```python
from build123d import *

# Parameters (mm, degrees)
BOSS_EXTRU_1_DEPTH        = 13
COQUE1_T                  = -5
COQUE1_THICKNESS_2_FACE_W = 65
COQUE1_THICKNESS_2_FACE_H = 65
COQUE1_THICKNESS_2_DEPTH  = 2
ENL_V_MAT_EXTRU_1_REACH   = 88.587
ESQUISSE2_R               = 2.5
ENL_V_MAT_EXTRU_2_REACH   = 95.396
ESQUISSE3_R               = 2.5
BOSS_EXTRU_2_DEPTH        = 10


with BuildPart() as part:
    # Esquisse1 → Boss.-Extru.1 (new body)
    with BuildSketch(Plane.XY):
        Polygon((44.118436308, 33.728448276), (54.118436308, 33.728448276), (54.118436308, 23.728448276), (54.118436308, -41.271551724), (-20.881563692, -41.271551724), (-20.881563692, 33.728448276), align=None)
    extrude(amount=BOSS_EXTRU_1_DEPTH)

    # Coque1
    coque1_openings = [part.faces().sort_by_distance(p)[0] for p in [
        (16.618436308, -3.771551724, 13),
    ]]
    offset(amount=COQUE1_T, openings=coque1_openings, kind=Kind.INTERSECTION)

    # Coque1 thickness 2 face (on inner face of the shell) → Coque1 thickness 2 (cut)
    with BuildSketch(Plane(origin=(16.618436308, -3.771551724, 5), x_dir=(-1, 0, 0), z_dir=(0, 0, -1))):
        Rectangle(COQUE1_THICKNESS_2_FACE_W, COQUE1_THICKNESS_2_FACE_H)
    extrude(amount=COQUE1_THICKNESS_2_DEPTH, mode=Mode.SUBTRACT)

    # Enlèv. mat.-Extru.1: up to this face of the body (flat: up to its plane)
    enl_v_mat_extru_1_end = Plane(part.part.faces().sort_by_distance((54.118436308, -3.771551724, 6.5))[0])
    # Esquisse2 → Enlèv. mat.-Extru.1 (cut, up to the picked face)
    with BuildSketch(Plane.ZY.offset(20.881563692), mode=Mode.PRIVATE) as enl_v_mat_extru_1_sk1:
        with Locations(Location((8, -16.271551724, 0), (0, 0, 270))):
            Circle(ESQUISSE2_R)
    enl_v_mat_extru_1_tool1 = split(extrude(enl_v_mat_extru_1_sk1.sketch, amount=-ENL_V_MAT_EXTRU_1_REACH, mode=Mode.PRIVATE), bisect_by=enl_v_mat_extru_1_end, keep=Keep.BOTH, mode=Mode.PRIVATE)
    # Esquisse2 → Enlèv. mat.-Extru.1 (cut, up to the picked face)
    with BuildSketch(Plane.ZY.offset(20.881563692), mode=Mode.PRIVATE) as enl_v_mat_extru_1_sk2:
        with Locations(Location((8, 8.728448276, 0), (0, 0, 270))):
            Circle(ESQUISSE2_R)
    enl_v_mat_extru_1_tool2 = split(extrude(enl_v_mat_extru_1_sk2.sketch, amount=-ENL_V_MAT_EXTRU_1_REACH, mode=Mode.PRIVATE), bisect_by=enl_v_mat_extru_1_end, keep=Keep.BOTH, mode=Mode.PRIVATE)
    add(enl_v_mat_extru_1_tool1.solids().sort_by(Axis((-20.881564, -16.271552, 8), (1, 0, 0)))[0], mode=Mode.SUBTRACT)
    add(enl_v_mat_extru_1_tool2.solids().sort_by(Axis((-20.881564, 8.728448, 8), (1, 0, 0)))[0], mode=Mode.SUBTRACT)

    # Enlèv. mat.-Extru.2: up to this face of the body (flat: up to its plane)
    enl_v_mat_extru_2_end = Plane(part.part.faces().sort_by_distance((16.618436308, 33.728448276, 6.5))[0])
    # Esquisse3 → Enlèv. mat.-Extru.2 (cut, up to the picked face)
    with BuildSketch(Plane.XZ.offset(41.271551724), mode=Mode.PRIVATE) as enl_v_mat_extru_2_sk1:
        with Locations(Location((4.118436308, 8, 0), (0, 0, 270))):
            Circle(ESQUISSE3_R)
    enl_v_mat_extru_2_tool1 = split(extrude(enl_v_mat_extru_2_sk1.sketch, amount=-ENL_V_MAT_EXTRU_2_REACH, mode=Mode.PRIVATE), bisect_by=enl_v_mat_extru_2_end, keep=Keep.BOTH, mode=Mode.PRIVATE)
    # Esquisse3 → Enlèv. mat.-Extru.2 (cut, up to the picked face)
    with BuildSketch(Plane.XZ.offset(41.271551724), mode=Mode.PRIVATE) as enl_v_mat_extru_2_sk2:
        with Locations(Location((29.118436308, 8, 0), (0, 0, 270))):
            Circle(ESQUISSE3_R)
    enl_v_mat_extru_2_tool2 = split(extrude(enl_v_mat_extru_2_sk2.sketch, amount=-ENL_V_MAT_EXTRU_2_REACH, mode=Mode.PRIVATE), bisect_by=enl_v_mat_extru_2_end, keep=Keep.BOTH, mode=Mode.PRIVATE)
    add(enl_v_mat_extru_2_tool1.solids().sort_by(Axis((4.118436, -41.271552, 8), (0, 1, 0)))[0], mode=Mode.SUBTRACT)
    add(enl_v_mat_extru_2_tool2.solids().sort_by(Axis((29.118436, -41.271552, 8), (0, 1, 0)))[0], mode=Mode.SUBTRACT)

    # Esquisse4 → Boss.-Extru.2 (add)
    with BuildSketch(Plane.XY.offset(3)):
        Polygon((-5.881563692, 28.728448276), (-15.881563692, 18.728448276), (-15.881563692, 28.728448276), align=None)
        Polygon((49.118436308, 28.728448276), (49.118436308, 18.728448276), (39.118436308, 28.728448276), align=None)
        Polygon((49.118436308, -36.271551724), (49.118436308, -26.271551724), (39.118436308, -36.271551724), align=None)
        Polygon((-5.881563692, -36.271551724), (-15.881563692, -26.271551724), (-15.881563692, -36.271551724), align=None)
    extrude(amount=BOSS_EXTRU_2_DEPTH)


solid = part.part
```
For this review, take the finished solid that the model builds, in its own axes (mm). A direction names the side the tool comes from. Coordinates: 2 decimals unless noted, no trailing zeros. Write each loop counter-clockwise with the first axis right and the second up, starting at its lowest first coordinate (ties: lowest second). Pieces come first, ordered by that corner, then holes. Notation, with made-up numbers: (59, 69.25) - (88, 69.25) arc R10 cw to (88, 74.25) - close; hole circle Ø4 at (-17, -34.5). An arc over 180 degrees is marked (long way). Put each result on its own line as item: value.
1. For pin 1 (6 mm diameter, centred on x = 17.5, y = -30.5, fed in from +Z), flat-tipped, find the tip position at first contact; note if it passes through.
Values found:
pin 1: z = 3
2. Wall thickness on probe 1 along X at (y, z) = (-38.15, 8); probe 2 along X at (y, z) = (-11, 12); probe 3 along Y at (x, z) = (9, 4.75): over which ranges is each line inside the solid? List them lowest first.
Values found:
probe 1: -20.88 to 1.62, 6.62 to 26.62, 31.62 to 54.12
probe 2: -20.88 to -15.88, 49.12 to 54.12
probe 3: -41.27 to -36.27, 28.73 to 33.73
3. Machinability: for faces 1 (the flat face through (44.188, 23.658, 7.93)), 2 (the flat face through (54.118, -4, 6)), which of the approach directions +Z, -Z, +X, -X, +Y, -Y give a long, thin tool a straight path to every point of the face, cutting with its end or side? Answer none if there is none.
Values found:
face 1: +Z
face 2: +Z, -Z, +X, +Y, -Y
4. Add section B-B, the plane z = 12. Give the boundary of the cut face in (x, y).
Values found:
outline: (-20.88, -41.27) - (54.12, -41.27) - (54.12, 33.73) - (-20.88, 33.73) - close; hole (-15.88, -26.27) - (-5.88, -36.27) - (39.12, -36.27) - (49.12, -26.27) - (49.12, 18.73) - (39.12, 28.73) - (-5.88, 28.73) - (-15.88, 18.73) - close
5. Add section A-A, the plane x = 18.5. Give the boundary of the cut face in (y, z).
Values found:
outline: (-41.27, 0) - (33.73, 0) - (33.73, 13) - (28.73, 13) - (28.73, 3) - (-36.27, 3) - (-36.27, 13) - (-41.27, 13) - close
6. Add section C-C, the plane y = 13. Give the boundary of the cut face in (x, z), then the cut area to 3 significant figures.
Values found:
outline: (-20.88, 0) - (54.12, 0) - (54.12, 13) - (49.12, 13) - (49.12, 3) - (-15.88, 3) - (-15.88, 13) - (-20.88, 13) - close
area: 325 mm²
7. Mouldability with a two-part tool opening along Y and no side actions: class faces 3 (the flat face through (17, -3, 3)), 4 (the flat face through (-20.882, -4, 6)), 5 (the flat face through (17, 33.728, 6)) as released by +Y, released by -Y, zero draft, split by the parting line, or undercut.
Values found:
face 3: undercut
face 4: zero draft
face 5: released by +Y
8. Add section D-D, the plane z = 8. Count the separate pieces of the cut face and the enclosed holes in it, then the cut area to 3 significant figures.
Values found:
separate pieces: 8
enclosed holes: 0
area: 1,400 mm²
